The figure shows three views and two pictorial views of one solid part (mm, origin at its lowest corner). Answer the questions. A direction names the side the tool comes from. Round coordinates to 2 decimals unless told otherwise and drop trailing zeros. Order: outer loops, then holes, each group sorted by start corner. A loop starts at its lowest first (then second) coordinate and runs counter-clockwise, first axis right, second up. Notation, with made-up numbers: (-8.75, 72.25) -> (47.25, 72.25) arc R25 cw to (47.25, 109.25) -> close; hole circle Ø3 at (61, -27). An arc over 180 degrees is marked (long way). Answer as a JSON object with one key per item and string values. Group by question number.
Item 1: For the marked faces 4, 5, 6 and 7, determine the directions among +Z, -Z, +X, -X, +Y, -Y from which every point of the face is accessible in a straight line to the end or side of a thin tool.
Item 2: Given P1, Ø2, axis at y = 96.5, z = 232, coming from the -X side; P2, Ø12, axis at y = 52.5, z = 200, coming from the +X side; P3, Ø3, axis at y = 129.5, z = 119, coming from the +X side (3 decimals), each flat-ended and moving along its own axis, determine where each tip first touches the part or whether it passes through.
Item 3: Consider probe 1 along Z at (x, y) = (127, 109); probe 2 along X at (y, z) = (112, 203); probe 3 along Y at (x, z) = (114.5, 85.5). Determine where each line is inside the solid, lowest interval first. Write a range as from..to.
Item 4: Section B-B, the plane x = 127 is taken. Write down the section's boundary in (y, z), plus the area to 3 significant figures.
Item 5: Section D-D, the plane z = 196.5 is taken. Write down the section's boundary in (x, y), plus the area to 3 significant figures.
Item 6: Section A-A, the plane y = 38 is taken. Count the separate pieces of the cut face and the enclosed holes in it, plus the area to 3 significant figures.
Item 7: The mould has two halves that part along Z. Classify the marked faces 1, 2 and 3: pulls with the +Z half, pulls with the -Z half, needs draft (parallel to the pull), parting line crosses it, or undercut.
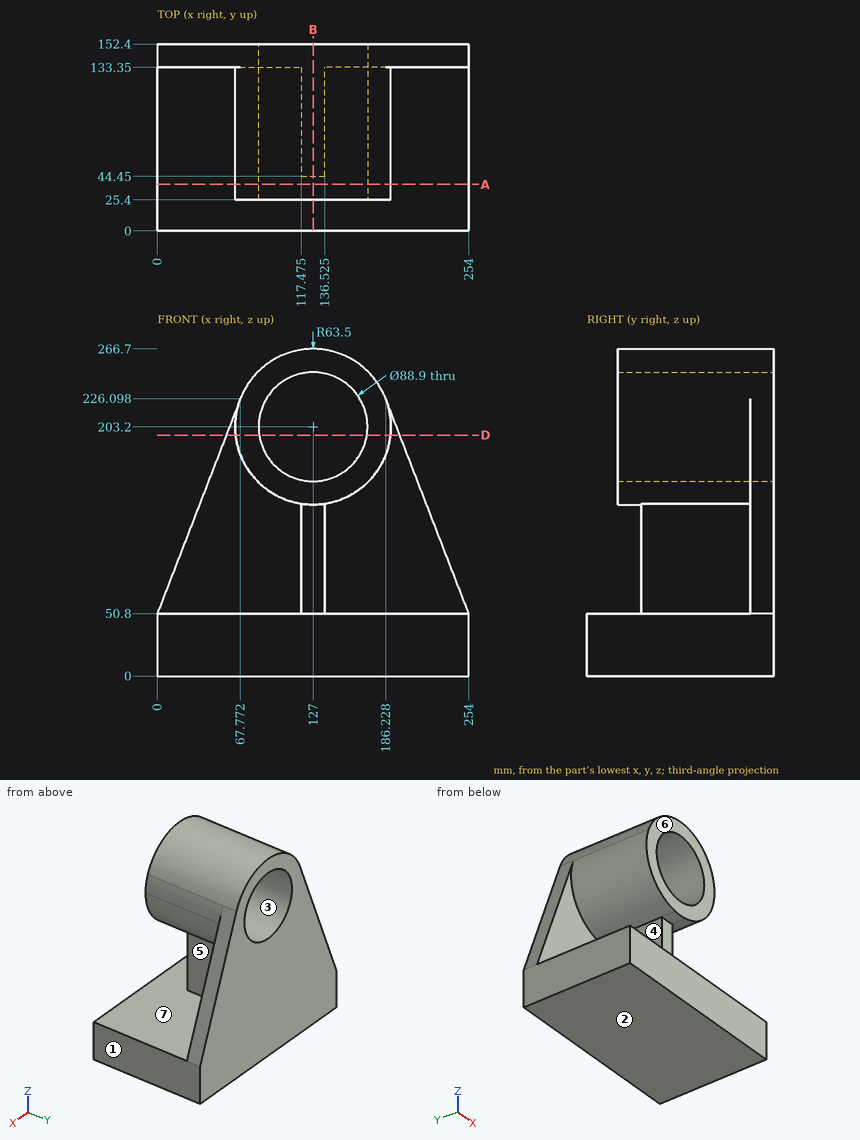
Values found:
{
 "1": {"face 4": "-X, -Y", "face 5": "+X, -Y", "face 6": "+Z, +X, -X, -Y", "face 7": "-Y"},
 "2": {"P1": "x = 69.91", "P2": "x = 190.5", "P3": "x = 136.525"},
 "3": {"probe 1": "0..158.75, 247.65..266.7", "probe 2": "63.5..82.55, 171.45..190.5", "probe 3": "133.35..152.4"},
 "4": {"outline": "(0, 0) -> (152.4, 0) -> (152.4, 158.75) -> (25.4, 158.75) -> (25.4, 139.7) -> (44.45, 139.7) -> (44.45, 50.8) -> (0, 50.8) -> close; (25.4, 247.65) -> (152.4, 247.65) -> (152.4, 266.7) -> (25.4, 266.7) -> close", "area": "22,200 mm2"},
 "5": {"outline": "(56.33, 133.35) -> (63.85, 133.35) -> (63.85, 25.4) -> (83.06, 25.4) -> (83.06, 152.4) -> (56.33, 152.4) -> close; (170.94, 25.4) -> (190.15, 25.4) -> (190.15, 133.35) -> (197.67, 133.35) -> (197.67, 152.4) -> (170.94, 152.4) -> close", "area": "5,160 mm2"},
 "6": {"separate pieces": "2", "enclosed holes": "1", "area": "19,400 mm2"},
 "7": {"face 1": "needs draft", "face 2": "pulls with the -Z half", "face 3": "undercut"}
}
